```python
from build123d import *

# Parameters (mm, degrees)
SKETCH1_W                    = 30
SKETCH1_H                    = 300
BASE_FLANGE1_DEPTH           = 2
EDGE_FLANGE1_STRIP_W         = 10
EDGE_FLANGE1_STRIP_H         = 2
EDGE_FLANGE1_STRIP_CUT_DEPTH = 300
EDGE_FLANGE1_DEPTH           = 300
CUT_EXTRUDE1_REACH           = 419.843
SKETCH8_W                    = 80
SKETCH8_H                    = 4.4
FILLET1_R                    = 1.5


# Sheet-metal steps are written as plain solids
with BuildPart() as part:
    # Sketch1 → Base-Flange1 (new body)
    with BuildSketch(Plane(origin=(0, -95.475928118, 0), x_dir=(1, 0, 0), z_dir=(0, 1, 0))):
        with Locations((-31.886491489, -255.528293106)):
            Rectangle(SKETCH1_W, SKETCH1_H)
    extrude(amount=BASE_FLANGE1_DEPTH)

    # Edge-Flange1 strip (across the edge) → Edge-Flange1 strip cut (cut)
    with BuildSketch(Plane(origin=(-16.886491489, -93.475928118, 405.528293106), x_dir=(-1, 0, 0), z_dir=(0, 0, -1))):
        with Locations((-4, -1)):
            Rectangle(EDGE_FLANGE1_STRIP_W, EDGE_FLANGE1_STRIP_H)
    extrude(amount=EDGE_FLANGE1_STRIP_CUT_DEPTH, mode=Mode.SUBTRACT)

    # Edge-Flange1 section (across the edge) → Edge-Flange1 (add)
    with BuildSketch(Plane(origin=(-16.886491489, -93.475928118, 405.528293106), x_dir=(-1, 0, 0), z_dir=(0, 0, -1))):
        with BuildLine():
            Line((-2, 1), (-2, 58))
            Line((-2, 58), (0, 58))
            Line((0, 58), (0, 1))
            ThreePointArc((0, 1), (0.292893219, 0.292893219), (1, 0))
            Line((1, 0), (1, -2))
            ThreePointArc((1, -2), (-1.121320344, -1.121320344), (-2, 1))
        make_face()
    extrude(amount=EDGE_FLANGE1_DEPTH)

    # Sketch8 → Cut-Extrude1 (cut, up to next)
    with BuildSketch(Plane(origin=(-14.886491489, 0, 0), x_dir=(0, 0, -1), z_dir=(1, 0, 0)), mode=Mode.PRIVATE) as cut_extrude1_sk1:
        with Locations((-160.528293106, -43.175928118)):
            Rectangle(SKETCH8_W, SKETCH8_H)
    cut_extrude1_tool1 = extrude(cut_extrude1_sk1.sketch, amount=-CUT_EXTRUDE1_REACH, mode=Mode.PRIVATE) & part.part
    # Sketch8 → Cut-Extrude1 (cut, up to next)
    with BuildSketch(Plane(origin=(-14.886491489, 0, 0), x_dir=(0, 0, -1), z_dir=(1, 0, 0)), mode=Mode.PRIVATE) as cut_extrude1_sk2:
        with Locations((-160.528293106, -59.175928118)):
            Rectangle(SKETCH8_W, SKETCH8_H)
    cut_extrude1_tool2 = extrude(cut_extrude1_sk2.sketch, amount=-CUT_EXTRUDE1_REACH, mode=Mode.PRIVATE) & part.part
    # Sketch8 → Cut-Extrude1 (cut, up to next)
    with BuildSketch(Plane(origin=(-14.886491489, 0, 0), x_dir=(0, 0, -1), z_dir=(1, 0, 0)), mode=Mode.PRIVATE) as cut_extrude1_sk3:
        with Locations((-350.528293106, -43.175928118)):
            Rectangle(SKETCH8_W, SKETCH8_H)
    cut_extrude1_tool3 = extrude(cut_extrude1_sk3.sketch, amount=-CUT_EXTRUDE1_REACH, mode=Mode.PRIVATE) & part.part
    # Sketch8 → Cut-Extrude1 (cut, up to next)
    with BuildSketch(Plane(origin=(-14.886491489, 0, 0), x_dir=(0, 0, -1), z_dir=(1, 0, 0)), mode=Mode.PRIVATE) as cut_extrude1_sk4:
        with Locations((-350.528293106, -59.175928118)):
            Rectangle(SKETCH8_W, SKETCH8_H)
    cut_extrude1_tool4 = extrude(cut_extrude1_sk4.sketch, amount=-CUT_EXTRUDE1_REACH, mode=Mode.PRIVATE) & part.part
    add(cut_extrude1_tool1.solids().sort_by_distance((-14.886491, -43.175928, 160.528293))[0], mode=Mode.SUBTRACT)
    add(cut_extrude1_tool2.solids().sort_by_distance((-14.886491, -59.175928, 160.528293))[0], mode=Mode.SUBTRACT)
    add(cut_extrude1_tool3.solids().sort_by_distance((-14.886491, -43.175928, 350.528293))[0], mode=Mode.SUBTRACT)
    add(cut_extrude1_tool4.solids().sort_by_distance((-14.886491, -59.175928, 350.528293))[0], mode=Mode.SUBTRACT)

    # Fillet1
    fillet1_edges = [part.edges().sort_by_distance(p)[0] for p in [
        (-15.886491489, -40.975928118, 120.528293106),
        (-15.886491489, -45.375928118, 120.528293106),
        (-15.886491489, -45.375928118, 200.528293106),
        (-15.886491489, -40.975928118, 200.528293106),
        (-15.886491489, -56.975928118, 120.528293106),
        (-15.886491489, -61.375928118, 120.528293106),
        (-15.886491489, -61.375928118, 200.528293106),
        (-15.886491489, -56.975928118, 200.528293106),
        (-15.886491489, -45.375928118, 390.528293106),
        (-15.886491489, -40.975928118, 390.528293106),
        (-15.886491489, -40.975928118, 310.528293106),
        (-15.886491489, -45.375928118, 310.528293106),
        (-15.886491489, -61.375928118, 390.528293106),
        (-15.886491489, -56.975928118, 390.528293106),
        (-15.886491489, -56.975928118, 310.528293106),
        (-15.886491489, -61.375928118, 310.528293106),
    ]]
    fillet(fillet1_edges, radius=FILLET1_R)


solid = part.part
```
The model under review builds one solid part; all positions refer to its coordinate system, in mm. A direction names the side the tool comes from. Round coordinates to 2 decimals unless told otherwise and drop trailing zeros. Order: outer loops, then holes, each group sorted by start corner. A loop starts at its lowest first (then second) coordinate and runs counter-clockwise, first axis right, second up.
Item 1: For pin 1 (3 mm diameter, centred on x = -37, z = 199, fed in from +Y); pin 2 (3 mm diameter, centred on y = -82, z = 271.5, fed in from -X); pin 3 (0.6 mm diameter, centred on x = -16, z = 158.5, fed in from -Y), all flat-tipped, find the tip position at first contact; note any pin that passes through.
Working result:
pin 1: stops at y = -93.48
pin 2: stops at x = -16.89
pin 3: stops at y = -95.02
Item 2: Machinability: for faces 1 (the flat face through (-16.7, -74.2, 105.528)), 2 (the flat face through (-33, -93.476, 253)), which of the approach directions +Z, -Z, +X, -X, +Y, -Y give a long, thin tool a straight path to every point of the face, cutting with its end or side? Answer none if there is none.
Working result:
face 1: -Z, +X, -X, +Y, -Y
face 2: +Z, -Z, -X, +Y
Item 3: Add section B-B, the plane z = 208.5. State the section outline as (x, y) points, and give its area (3 significant figures).
Working result:
outline: (-46.89, -95.48) - (-17.89, -95.48) arc R3 ccw to (-14.89, -92.48) - (-14.89, -35.48) - (-16.89, -35.48) - (-16.89, -92.48) arc R1 cw to (-17.89, -93.48) - (-46.89, -93.48) - close
area: 178 mm2
Item 4: Add section C-C, the plane x = -24.5. State the section outline as (y, z) points, and give its area (3 significant figures).
Working result:
outline: (-95.48, 105.53) - (-93.48, 105.53) - (-93.48, 405.53) - (-95.48, 405.53) - close
area: 600 mm2
Item 5: Add section D-D, the plane y = -85.5. State the section outline as (x, z) points.
Working result:
outline: (-16.89, 105.53) - (-14.89, 105.53) - (-14.89, 405.53) - (-16.89, 405.53) - close
Item 6: To check wall thickness, follow probe 1 along X at (y, z) = (-54, 168); probe 2 along Y at (x, z) = (-24, 302); probe 3 along Y at (x, z) = (-17, 164.5). State the ranges of each line that lie inside material, in increasing order.
Working result:
probe 1: x = -16.89 to -14.89
probe 2: y = -95.48 to -93.48
probe 3: y = -95.34 to -92.94
Item 7: Add section A-A, the plane z = 169.5. State the section outline as (x, y) points, and give its area (3 significant figures).
Working result:
outline: (-46.89, -95.48) - (-17.89, -95.48) arc R3 ccw to (-14.89, -92.48) - (-14.89, -61.38) - (-16.89, -61.38) - (-16.89, -92.48) arc R1 cw to (-17.89, -93.48) - (-46.89, -93.48) - close; (-16.89, -56.98) - (-14.89, -56.98) - (-14.89, -45.38) - (-16.89, -45.38) - close; (-16.89, -40.98) - (-14.89, -40.98) - (-14.89, -35.48) - (-16.89, -35.48) - close
area: 161 mm2
